from build123d import *

# Parameters (mm, degrees)
F1_DEPTH = 150
F2_SIZE  = 22
F3_R     = 15
F4_DEPTH = 25


with BuildPart() as f1:
    # F0 (on Top) → F1 (new body)
    with BuildSketch(Plane.XY):
        Polygon((-70, 0), (0, 0), (0, 70), (-7, 70), (-7, 7), (-70, 7), align=None)
    extrude(amount=F1_DEPTH)

    # F2
    f2_edges = [f1.edges().sort_by_distance(p)[0] for p in [
        (-70, 3.5, 150),
        (-3.5, 70, 150),
    ]]
    chamfer(f2_edges, length=F2_SIZE)

    # F3 (on face) → F4 (cut)
    with BuildSketch(Plane.YZ):
        with Locations((35, 115)):
            Circle(F3_R)
    extrude(amount=-F4_DEPTH, mode=Mode.SUBTRACT)


solid = f1.part
Read the model definition and answer for the solid it produces. Units are mm, in the model's axes. A direction names the side the tool comes from. Coordinates: 2 decimals unless noted, no trailing zeros. Loops run counter-clockwise (first coordinate to the right, second up) from the corner with the lowest first, then second, coordinate; pieces in that order, holes last. Notation, with made-up numbers: (58.5, 26) - (87.5, 26) arc R12 cw to (87.5, 45) - close; hole circle Ø1 at (12.25, -38). An arc over 180 degrees is marked (long way). Answer in a Markdown table with one row per item.
Q1. Find section C-C on x = -5. Write down the section's boundary in (y, z).
Here are the results:
| item | result |
|---|---|
| outline | (0, 0) - (70, 0) - (70, 128) - (48, 150) - (0, 150) - close; hole circle Ø30 at (35, 115) |
Q2. The mould has two halves that part along Y. Classify faces 1 (the cylindrical face through (-3.451, 23.944, 125.138)), 2 (the flat face through (-3, 59, 139)), 3 (the flat face through (-35, 0, 74)), 4 (the flat face through (0, 35, 74)): pulls with the +Y half, pulls with the -Y half, needs draft (parallel to the pull), parting line crosses it, or undercut.
Here are the results:
| item | result |
|---|---|
| face 1 | undercut |
| face 2 | pulls with the +Y half |
| face 3 | pulls with the -Y half |
| face 4 | needs draft |
Q3. For faces 5 (the flat face through (-38, 7, 74)), 6 (the flat face through (-70, 4, 63)), determine the directions among +Z, -Z, +X, -X, +Y, -Y from which every point of the face is accessible in a straight line to the end or side of a thin tool.
Here are the results:
| item | result |
|---|---|
| face 5 | +Z, -Z, -X, +Y |
| face 6 | +Z, -Z, -X, +Y, -Y |
Q4. Find section B-B on y = 35. Write down the section's boundary in (x, z), plus the area to 3 significant figures.
Here are the results:
| item | result |
|---|---|
| outline | (-7, 0) - (0, 0) - (0, 100) - (-7, 100) - close; (-7, 130) - (0, 130) - (0, 150) - (-7, 150) - close |
| area | 840 mm^2 |
Q5. Find section D-D on z = 77.5. Write down the section's boundary in (x, y).
Here are the results:
| item | result |
|---|---|
| outline | (-70, 0) - (0, 0) - (0, 70) - (-7, 70) - (-7, 7) - (-70, 7) - close |
Q6. Find section A-A on z = 115. Write down the section's boundary in (x, y).
Here are the results:
| item | result |
|---|---|
| outline | (-70, 0) - (0, 0) - (0, 20) - (-7, 20) - (-7, 7) - (-70, 7) - close; (-7, 50) - (0, 50) - (0, 70) - (-7, 70) - close |
Q7. Given P1, Ø8, axis at x = -61.5, z = 47, coming from the -Y side; P2, Ø2, axis at x = -54.5, z = 65, coming from the +Y side; P3, Ø24, axis at y = 35, z = 115, coming from the -X side; P4, Ø5, axis at y = 30.5, z = 88.5, coming from the -X side, each flat-ended and moving along its own axis, determine where each tip first touches the part or whether it passes through.
Here are the results:
| item | result |
|---|---|
| P1 | stops at y = 0 |
| P2 | stops at y = 7 |
| P3 | passes through |
| P4 | stops at x = -7 |
Q8. Straight lines are drawn through the part: line 1 along Z through (x, y) = (-4, 35); line 2 along X through (y, z) = (55.5, 139.5); line 3 along Y through (x, z) = (-32.5, 103). For each, find the intervals that lie inside material, in ascending order. Write a range as [from, to].
Here are the results:
| item | result |
|---|---|
| line 1 | z = [0, 100], [130, 150] |
| line 2 | x = [-7, 0] |
| line 3 | y = [0, 7] |
